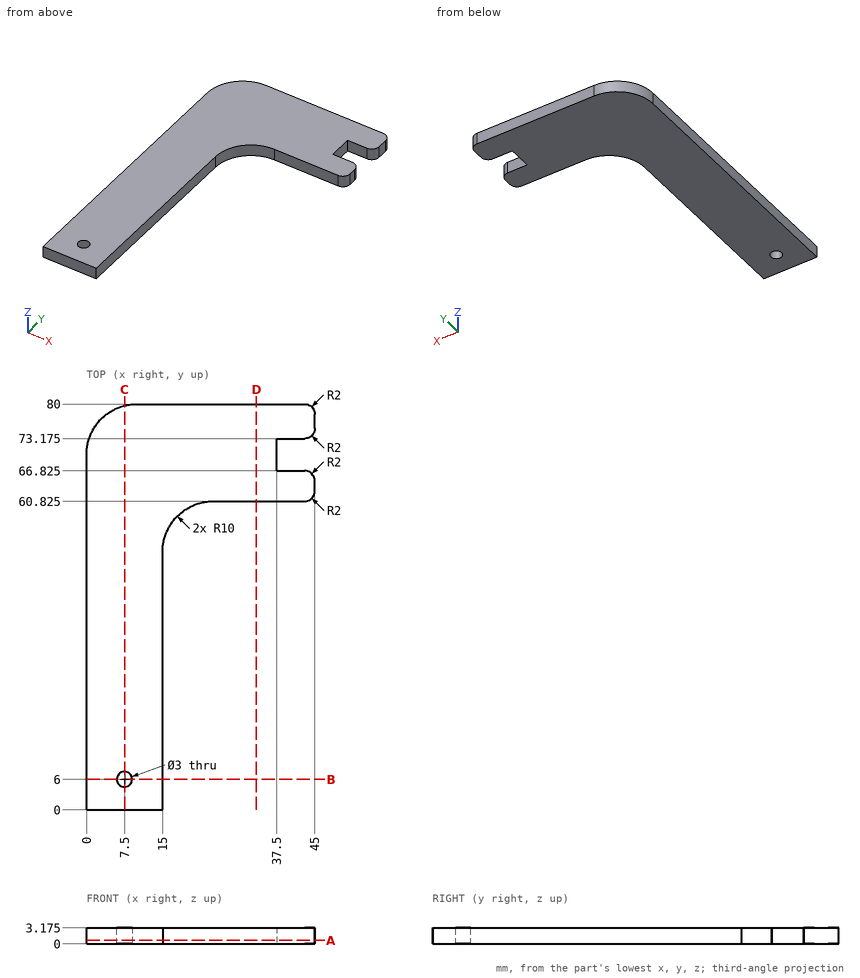
The drawing under review shows one solid part. Ordinate dimensions are in mm from its lowest x, y, z. Coordinates: 2 decimals unless noted, no trailing zeros. Write each loop counter-clockwise with the first axis right and the second up, starting at its lowest first coordinate (ties: lowest second). Pieces come first, ordered by that corner, then holes. Notation, with made-up numbers: (-25, -29) - (-18, -29) arc R7 cw to (-18, -24) - close; hole circle Ø2 at (6.5, 0.5). An arc over 180 degrees is marked (long way). Answer in a Markdown table with one row per item. Add a question column.
Q1. We need section A-A, the plane z = 0.7. State the section outline as (x, y) points (3 decimals), and give its area (3 significant figures).
Q2. We need section C-C, the plane x = 7.5. State the section outline as (y, z) points (3 decimals), and give its area (3 significant figures).
Q3. For probe 1 along X at (y, z) = (6, 1.35); probe 2 along X at (y, z) = (28, 1.85); probe 3 along Y at (x, z) = (34.5, 2.75) (3 decimals), list the stretches that pass through material, from the lowest coordinate up.
Q4. We need section B-B, the plane y = 6. State the section outline as (x, z) points (3 decimals).
Q5. For P1, Ø1, axis at y = 71, z = 1.5, coming from the -X side; P2, Ø1.6, axis at y = 31, z = 1.5, coming from the +X side; P3, Ø1.5, axis at y = 66.5, z = 2.5, coming from the +X side, all flat-tipped, find the tip position at first contact; note any pin that passes through.
Q6. We need section D-D, the plane x = 33.5. State the section outline as (y, z) points (3 decimals), and give its area (3 significant figures).
Answer list:
| question | item | result |
|---|---|---|
| 1 | outline | (0, 0) - (15, 0) - (15, 50.825) arc R10 cw to (25, 60.825) - (43, 60.825) arc R2 ccw to (45, 62.825) - (45, 64.825) arc R2 ccw to (43, 66.825) - (37.5, 66.825) - (37.5, 73.175) - (43, 73.175) arc R2 ccw to (45, 75.175) - (45, 78) arc R2 ccw to (43, 80) - (10, 80) arc R10 ccw to (0, 70) - close; hole circle Ø3 at (7.5, 6) |
| 1 | area | 1,720 mm2 |
| 2 | outline | (0, 0) - (4.5, 0) - (4.5, 3.175) - (0, 3.175) - close; (7.5, 0) - (79.682, 0) - (79.682, 3.175) - (7.5, 3.175) - close |
| 2 | area | 243 mm2 |
| 3 | probe 1 | x = 0 to 6, 9 to 15 |
| 3 | probe 2 | x = 0 to 15 |
| 3 | probe 3 | y = 60.825 to 80 |
| 4 | outline | (0, 0) - (6, 0) - (6, 3.175) - (0, 3.175) - close; (9, 0) - (15, 0) - (15, 3.175) - (9, 3.175) - close |
| 5 | P1 | stops at x = 0.01 |
| 5 | P2 | stops at x = 15 |
| 5 | P3 | stops at x = 44.77 |
| 6 | outline | (60.825, 0) - (80, 0) - (80, 3.175) - (60.825, 3.175) - close |
| 6 | area | 60.9 mm2 |
